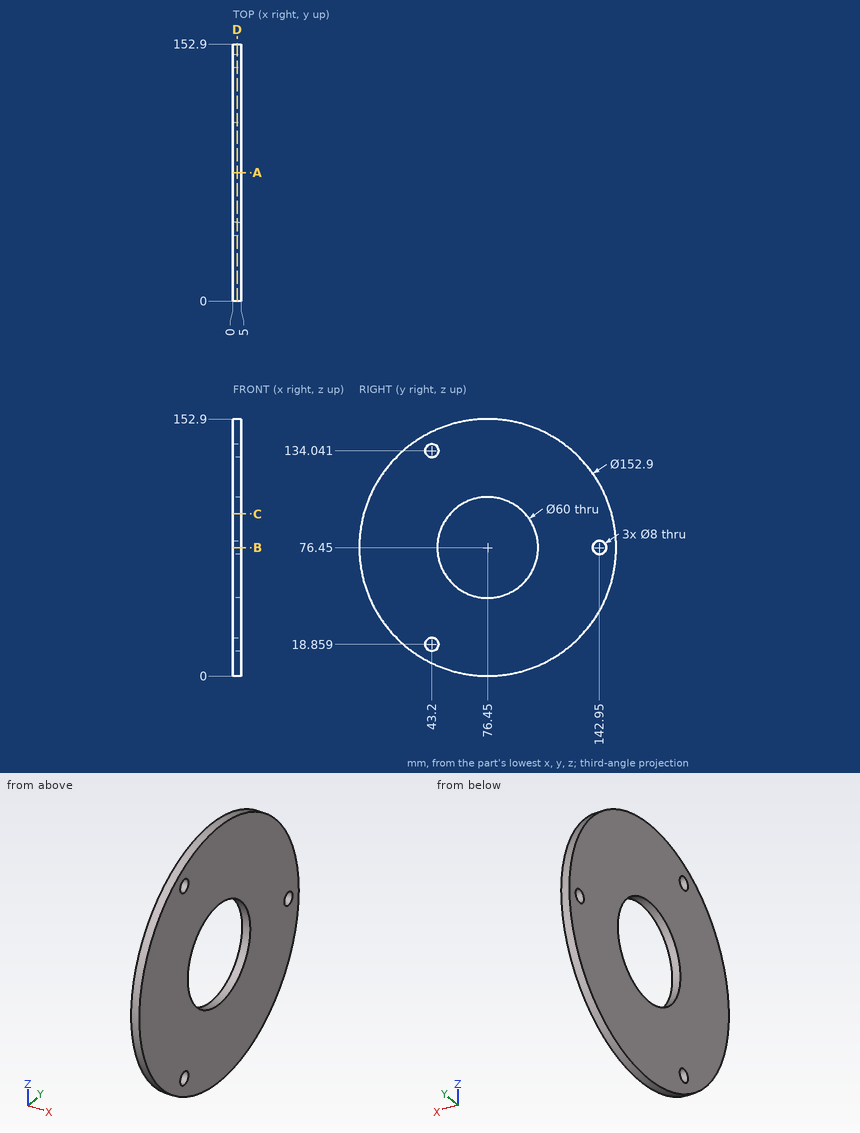
Geometry check sheet. Reference: drawing and pictorial views, mm from the part's lowest x, y, z. Give positions to 0.01 mm unless a question says otherwise; leave off trailing zeros. Loops run counter-clockwise (first coordinate to the right, second up) from the corner with the lowest first, then second, coordinate; pieces in that order, holes last. Notation, with made-up numbers: M 58.25,38.25 L 67.25,38.25 A22 cw 67.25,56.25 Z; hole C 50.25,50.5 d2. An arc over 180 degrees is marked long. Use a Markdown table: item, result. Add a question column.
Q1. Sectioned sample at A-A, the plane y = 76.45. Record the cut outline in (x, z).
Q2. Sectioned sample at C-C, the plane z = 96.5. Record the cut outline in (x, y).
Q3. Sectioned sample at D-D, the plane x = 2.55. Record the cut outline in (y, z), then the cut area to 3 significant figures.
Q4. Scan lines: line 1 along Y through (x, z) = (4.25, 80) (1 decimal); line 2 along Z through (x, y) = (1.2, 76.45); line 3 along Z through (x, y) = (3.6, 43.2). Record each from-to range of solid material in increasing order. Write a range as [from, to].
Q5. Go/stop test with flat-tipped pins: pin 1 (7 mm diameter, centred on y = 142.95, z = 76.45, fed in from +X); pin 2 (1 mm diameter, centred on x = 4.5, y = 136.5, fed in from +Z); pin 3 (1 mm diameter, centred on x = 2, y = 87, fed in from +Z). Record where each tip stops, or that it passes through.
Q6. Sectioned sample at B-B, the plane z = 76.45. Record the cut outline in (x, y).
Verdict:
| question | item | result |
|---|---|---|
| 1 | outline | M 0,0 L 5,0 L 5,46.45 L 0,46.45 Z; M 0,106.45 L 5,106.45 L 5,152.9 L 0,152.9 Z |
| 2 | outline | M 0,2.68 L 5,2.68 L 5,54.13 L 0,54.13 Z; M 0,98.77 L 5,98.77 L 5,150.22 L 0,150.22 Z |
| 3 | outline | C 76.45,76.45 d152.9; hole C 43.2,18.86 d8; hole C 43.2,134.04 d8; hole C 76.45,76.45 d60; hole C 142.95,76.45 d8 |
| 3 | area | 15,400 mm^2 |
| 4 | line 1 | [0.1, 46.7], [106.2, 141.1], [144.8, 152.8] |
| 4 | line 2 | [0, 46.45], [106.45, 152.9] |
| 4 | line 3 | [7.61, 14.86], [22.86, 130.04], [138.04, 145.29] |
| 5 | pin 1 | through |
| 5 | pin 2 | z = 124.39 |
| 5 | pin 3 | z = 152.24 |
| 6 | outline | M 0,0 L 5,0 L 5,46.45 L 0,46.45 Z; M 0,106.45 L 5,106.45 L 5,138.95 L 0,138.95 Z; M 0,146.95 L 5,146.95 L 5,152.9 L 0,152.9 Z |
